```python
from build123d import *

# Parameters (mm, degrees)
F0_R     = 5
F1_DEPTH = 10
F2_R     = 10
F3_R     = 1
F4_DEPTH = 6
F5_R     = 1.99999
F6_R     = 2


# Not quite as in the source:
# - a fillet or chamfer is up to 0.001 mm smaller than in the source, because OpenCascade refuses the exact size


with BuildPart() as f1:
    # F0 (on Top) → F1 (new body)
    with BuildSketch(Plane.XY):
        with BuildLine():
            ThreePointArc((87.8922518749, 12.982062427), (61.2373823548, 18.6986926605), (39.2710061569, 34.8430491695))
            ThreePointArc((39.2710061569, 34.8430491695), (-52.4855584858, 1.231320604), (37.5938529252, -36.6463125326))
            ThreePointArc((37.5938529252, -36.6463125326), (58.881501719, -22.1257192654), (84.1386232135, -17.017937573))
            Line((84.1386232135, -17.017937573), (188.9996444946, -17.017937573))
            Line((188.9996444946, -17.017937573), (188.9996444946, 12.982062427))
            Line((188.9996444946, 12.982062427), (87.8922518749, 12.982062427))
        make_face()
        with BuildLine():
            ThreePointArc((-28.0871828778, 24.8467333464), (-18.7727000217, 32.4628361961), (-7.5256854941, 36.7370937588))
            Line((-7.5256854941, 36.7370937588), (-7.6951050263, 31.7399648809))
            Line((-7.6951050263, 31.7399648809), (7.3048913079, 31.7504516883))
            Line((7.3048913079, 31.7504516883), (7.4743108401, 36.7475805661))
            ThreePointArc((7.4743108401, 36.7475805661), (18.7272908139, 32.4890532145), (28.0524137093, 24.8859816982))
            Line((28.0524137093, 24.8859816982), (23.6400633889, 22.5341388781))
            Line((23.6400633889, 22.5341388781), (31.1491433976, 9.5490043996))
            Line((31.1491433976, 9.5490043996), (35.561493718, 11.9008472197))
            ThreePointArc((35.561493718, 11.9008472197), (37.4999908356, 0.0262170183), (35.5780992034, -11.8511120606))
            Line((35.5780992034, -11.8511120606), (31.3351684153, -9.2058260029))
            Line((31.3351684153, -9.2058260029), (23.8442520897, -22.2014472886))
            Line((23.8442520897, -22.2014472886), (28.0871828778, -24.8467333464))
            ThreePointArc((28.0871828778, -24.8467333464), (18.7727000217, -32.4628361961), (7.5256854941, -36.7370937588))
            Line((7.5256854941, -36.7370937588), (7.6951050263, -31.7399648809))
            Line((7.6951050263, -31.7399648809), (-7.3048913079, -31.7504516883))
            Line((-7.3048913079, -31.7504516883), (-7.4743108401, -36.7475805661))
            ThreePointArc((-7.4743108401, -36.7475805661), (-18.7272908139, -32.4890532145), (-28.0524137093, -24.8859816982))
            Line((-28.0524137093, -24.8859816982), (-23.6400633889, -22.5341388781))
            Line((-23.6400633889, -22.5341388781), (-31.1491433976, -9.5490043996))
            Line((-31.1491433976, -9.5490043996), (-35.561493718, -11.9008472197))
            ThreePointArc((-35.561493718, -11.9008472197), (-37.4999908356, -0.0262170183), (-35.5780992034, 11.8511120606))
            Line((-35.5780992034, 11.8511120606), (-31.3351684153, 9.2058260029))
            Line((-31.3351684153, 9.2058260029), (-23.8442520897, 22.2014472886))
            Line((-23.8442520897, 22.2014472886), (-28.0871828778, 24.8467333464))
        make_face(mode=Mode.SUBTRACT)
        with BuildLine():
            Line((159.6448034048, -5), (59.6448034048, -5))
            ThreePointArc((59.6448034048, -5), (54.6448034048, 0), (59.6448034048, 5))
            Line((59.6448034048, 5), (159.6448034048, 5))
            ThreePointArc((159.6448034048, 5), (164.6448034048, 0), (159.6448034048, -5))
        make_face(mode=Mode.SUBTRACT)
        with Locations((176.5601634979, 0)):
            Circle(F0_R, mode=Mode.SUBTRACT)
    extrude(amount=F1_DEPTH)

    # F2
    f2_edges = [f1.edges().sort_by_distance(p)[0] for p in [
        (188.999644, 12.982062, 5),
        (188.999644, -17.017938, 5),
    ]]
    fillet(f2_edges, radius=F2_R)

    # F3
    f3_edges = [f1.edges().sort_by_distance(p)[0] for p in [
        (-7.525685, 36.737094, 5),
        (-7.695105, 31.739965, 5),
        (7.304891, 31.750452, 5),
        (7.474311, 36.747581, 5),
        (23.640063, 22.534139, 5),
        (28.052414, 24.885982, 5),
        (31.149143, 9.549004, 5),
        (35.561494, 11.900847, 5),
        (35.578099, -11.851112, 5),
        (31.335168, -9.205826, 5),
        (23.844252, -22.201447, 5),
        (28.087183, -24.846733, 5),
        (7.525685, -36.737094, 5),
        (7.695105, -31.739965, 5),
        (-7.304891, -31.750452, 5),
        (-7.474311, -36.747581, 5),
        (-28.052414, -24.885982, 5),
        (-23.640063, -22.534139, 5),
        (-31.149143, -9.549004, 5),
        (-35.561494, -11.900847, 5),
        (-35.578099, 11.851112, 5),
        (-31.335168, 9.205826, 5),
        (-23.844252, 22.201447, 5),
        (-28.087183, 24.846733, 5),
    ]]
    fillet(f3_edges, radius=F3_R)

    # F0 (on Top) → F4 (join)
    with BuildSketch(Plane.XY):
        with BuildLine():
            ThreePointArc((59.6448034048, 5), (54.6448034048, 0), (59.6448034048, -5))
            Line((59.6448034048, -5), (159.6448034048, -5))
            ThreePointArc((159.6448034048, -5), (164.6448034048, 0), (159.6448034048, 5))
            Line((159.6448034048, 5), (59.6448034048, 5))
        make_face()
    extrude(amount=F4_DEPTH)

    # F5 (radius 2 in the source; OpenCascade refuses exactly that, so slightly less here)
    f5_edges = [f1.edges().sort_by_distance(p)[0] for p in [
        (109.644803, 5, 6),
        (109.644803, 5, 10),
    ]]
    fillet(f5_edges, radius=F5_R)

    # F6
    f6_edges = [f1.edges().sort_by_distance(p)[0] for p in [
        (-52.485558, 1.231321, 10),
    ]]
    fillet(f6_edges, radius=F6_R)


solid = f1.part
```
The listing builds one solid part. Answer for the finished solid, in the listing's coordinates (mm). A direction names the side the tool comes from. Round coordinates to 2 decimals unless told otherwise and drop trailing zeros.
1) Given P1, Ø1.5, axis at x = 76, y = -1.5, coming from the +Z side; P2, Ø1, axis at x = 123.5, z = 6, coming from the -Y side; P3, Ø1.5, axis at y = 33.5, z = 4.5, coming from the +X side, each flat-ended and moving along its own axis, determine where each tip first touches the part or whether it passes through.
Outcome:
P1: stops at z = 6
P2: stops at y = -17.02
P3: stops at x = 41.21
2) Consider line 1 (Y direction, x = 87, z = 8); line 2 (Y direction, x = 116, z = 4); line 3 (Y direction, x = 150, z = 6.75). Determine where each line is inside the solid, lowest interval first.
Outcome:
line 1: y = -17.02 to -5, 5 to 12.99
line 2: y = -17.02 to 12.98
line 3: y = -17.02 to -4.56, 4.56 to 12.98
3) For faces 1 (the face through (-27.366, -16.09, 4.93)), 2 (the face through (131, -17.018, 4)), 3 (the face through (109, 0, 6)), determine the directions among +Z, -Z, +X, -X, +Y, -Y from which every point of the face is accessible in a straight line to the end or side of a thin tool.
Outcome:
face 1: +Z, -Z
face 2: +Z, -Z, +X, -Y
face 3: +Z
4) A cutting plane is placed at B-B on y = 0. Give the number of separate pieces and of enclosed holes in the cut face, plus the area to 3 significant figures.
Outcome:
separate pieces: 3
enclosed holes: 0
area: 1,120 mm2
5) For a pull along X with two mould halves and no side action, classify faces 4 (the face through (134, 12.982, 4)), 5 (the face through (-27.62, 15.65, 4.93)), 6 (the face through (18.556, 32.587, 4.93)), 7 (the face through (185.993, 10.13, 4.056)) as released by +X, released by -X, zero draft, split by the parting line, or undercut.
Outcome:
face 4: zero draft
face 5: undercut
face 6: undercut
face 7: released by +X
